Verification items for this drawing (mm, ordinates from the low corner). Give positions to 0.01 mm unless a question says otherwise; leave off trailing zeros. Loops run counter-clockwise (first coordinate to the right, second up) from the corner with the lowest first, then second, coordinate; pieces in that order, holes last. Notation, with made-up numbers: M -36,89 L 13,89 A18 ccw 13,106 Z; hole C 46,24 d11. An arc over 180 degrees is marked long. Use a Markdown table: item, result.
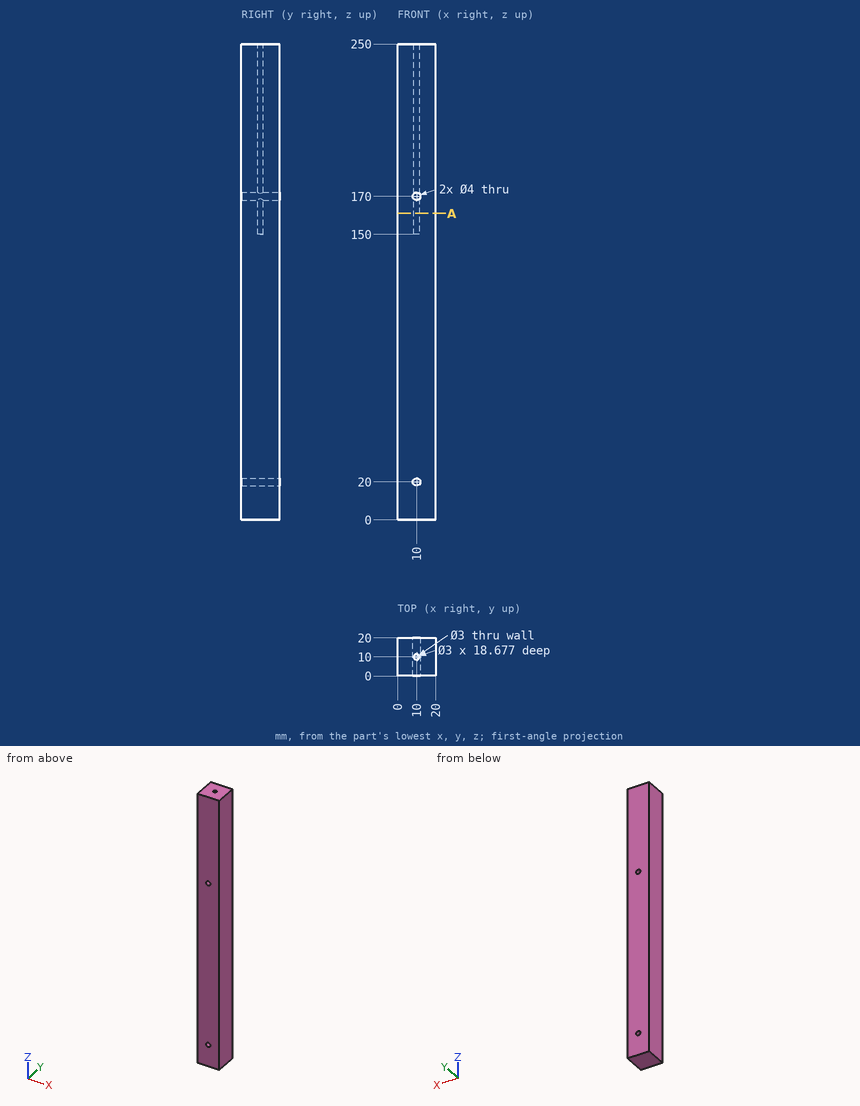
(1) Cross-section at A-A on z = 161. Record the cut outline in (x, y).
Results below:
| item | result |
|---|---|
| outline | M 0,0 L 20,0 L 20,20 L 0,20 Z; hole C 10,10 d3 |
(2) Material ranges on line 1 (Z direction, x = 10, y = 5); line 2 (X direction, y = 7, z = 20); line 3 (Y direction, x = 10, z = 205.5), recorded low to high.
Results below:
| item | result |
|---|---|
| line 1 | 0 to 18, 22 to 168, 172 to 250 |
| line 2 | 0 to 8, 12 to 20 |
| line 3 | 0 to 8.5, 11.5 to 20 |
(3) Gauge pin test, flat end, axial feed: P1, Ø2.5, axis at x = 10, y = 10, coming from the +Z side. Record the tip position at first contact, or that the pin passes through.
Results below:
| item | result |
|---|---|
| P1 | z = 150 |
